```python
from build123d import *

# Parameters (mm, degrees)
SKETCH1_W          = 10
SKETCH1_H          = 54
BASE_FLANGE1_DEPTH = 0.5
EDGE_FLANGE1_DEPTH = 54
CUT_EXTRUDE1_DEPTH = 10
EDGE_FLANGE2_DEPTH = 19.2634
SKETCH11_R         = 1.8
CUT_EXTRUDE2_DEPTH = 10
SKETCH12_R         = 2
CUT_EXTRUDE3_DEPTH = 10


# Sheet-metal steps are written as plain solids
with BuildPart() as part:
    # Sketch1 → Base-Flange1 (new body)
    with BuildSketch(Plane(origin=(0, 0, 0), x_dir=(1, 0, 0), z_dir=(0, 1, 0))):
        with Locations((-31.456172324, -6.536484397)):
            Rectangle(SKETCH1_W, SKETCH1_H)
    extrude(amount=-BASE_FLANGE1_DEPTH)

    # Edge-Flange1 section (across the edge) → Edge-Flange1 (add)
    with BuildSketch(Plane(origin=(-37.192772324, -0.5, 33.536484397), x_dir=(1, 0, 0), z_dir=(0, 0, -1))):
        with BuildLine():
            Line((-0.5, 0.7366), (-0.5, 20))
            Line((-0.5, 20), (0, 20))
            Line((0, 20), (0, 0.7366))
            ThreePointArc((0, 0.7366), (0.215745145, 0.215745145), (0.7366, 0))
            Line((0.7366, 0), (0.7366, -0.5))
            ThreePointArc((0.7366, -0.5), (-0.137808246, -0.137808246), (-0.5, 0.7366))
        make_face()
    extrude(amount=EDGE_FLANGE1_DEPTH)

    # Sketch7 → Cut-Extrude1 (cut)
    with BuildSketch(Plane.ZY.offset(37.692772324)):
        Polygon((-20.463515603, -20.5), (33.536484397, -1.2366), (33.536484397, -20.5), align=None)
    extrude(amount=-CUT_EXTRUDE1_DEPTH, mode=Mode.SUBTRACT)

    # Edge-Flange2 section (across the edge) → Edge-Flange2 (add)
    with BuildSketch(Plane(origin=(-37.192772324, -20.5, -21.200115603), x_dir=(0, 0, 1), z_dir=(0, 1, 0))):
        with BuildLine():
            Line((-0.5, 0.7366), (-0.5, 10))
            Line((-0.5, 10), (0, 10))
            Line((0, 10), (0, 0.7366))
            ThreePointArc((0, 0.7366), (0.215745145, 0.215745145), (0.7366, 0))
            Line((0.7366, 0), (0.7366, -0.5))
            ThreePointArc((0.7366, -0.5), (-0.137808246, -0.137808246), (-0.5, 0.7366))
        make_face()
    extrude(amount=EDGE_FLANGE2_DEPTH)

    # Sketch11 → Cut-Extrude2 (cut)
    with BuildSketch(Plane(origin=(0, 0, -21.700115603), x_dir=(-1, 0, 0), z_dir=(0, 0, -1))):
        with Locations((31.456172324, -6.2366)):
            Circle(SKETCH11_R)
        with Locations((31.456172324, -16.2366)):
            Circle(SKETCH11_R)
    extrude(amount=-CUT_EXTRUDE2_DEPTH, mode=Mode.SUBTRACT)

    # Sketch12 → Cut-Extrude3 (cut)
    with BuildSketch(Plane(origin=(0, 0, 0), x_dir=(1, 0, 0), z_dir=(0, 1, 0))):
        with Locations(Location((-32.456172324, -29.536484397, 0), (0, 0, 270))):
            Circle(SKETCH12_R)
        with Locations(Location((-32.456172324, 15.963515603, 0), (0, 0, 270))):
            Circle(SKETCH12_R)
    extrude(amount=-CUT_EXTRUDE3_DEPTH, mode=Mode.SUBTRACT)


solid = part.part
```
Design review of the part built by this model. Coordinates are the model's own, in mm. A direction names the side the tool comes from. Round coordinates to 2 decimals unless told otherwise and drop trailing zeros. Write each loop counter-clockwise with the first axis right and the second up, starting at its lowest first coordinate (ties: lowest second). Pieces come first, ordered by that corner, then holes. Notation, with made-up numbers: (78.25, 58.25) -> (108.25, 58.25) arc R21 ccw to (108.25, 70.25) -> close; hole circle Ø3 at (-11.75, 7). An arc over 180 degrees is marked (long way). Write item = value, one per line. Start each with the question number.
1) Tool access review of faces 1 (the face through (-37.193, -7, -5)), 2 (the face through (-32, -11, -21.2)), 3 (the face through (-32, -0.5, 6)), 4 (the face through (-32.4, -20.5, -21.5)), 5 (the face through (-37.446, -11.003, 6.158)): name each direction out of +Z, -Z, +X, -X, +Y, -Y from which nothing blocks a thin tool from reaching the whole face with its end or side.
2) Take a section at A-A, the plane x = -35.5. State the section outline as (y, z) points, plus the area to 3 significant figures.
3) Clearance check with flat-ended pins moving along their axes: pin 1 (3 mm diameter, centred on x = -32, z = -13.5, fed in from -Y); pin 2 (4.5 mm diameter, centred on x = -31.46, y = -6.24, fed in from +Z); pin 3 (3 mm diameter, centred on y = -3, z = -12, fed in from +X). State where each tip first meets the part, or that it passes through.
4) Take a section at D-D, the plane z = 11. State the section outline as (x, y) points, plus the area to 3 significant figures.
5) Wall thickness on probe 1 along Y at (x, z) = (-30, -16); probe 2 along X at (y, z) = (-1.5, -19); probe 3 along Z at (x, y) = (-31.5, -12): over which ranges is each line inside the solid? List them lowest first. Write a range as from..to.
6) Take a section at C-C, the plane y = -7. State the section outline as (x, z) points.
7) Mouldability with a two-part tool opening along Y and no side actions: class faces 6 (the face through (-32, 0, 6)), 7 (the face through (-29.658, -16.157, -21.454)), 8 (the face through (-37.34, -11, -21.33)), 9 (the face through (-29.658, -6.157, -21.454)) as +Y half, -Y half, draft (parallel to the pull), parting line (faces both ways), or undercut.
8) Take a section at B-B, the plane x = -31.5. State the section outline as (y, z) points, plus the area to 3 significant figures.
Results list:
q1.face_1 = +Z, +X, -Y
q1.face_2 = +Z, +X, +Y, -Y
q1.face_3 = +Z, -Z, +X, -Y
q1.face_4 = +Z, -Z, +X, -X, -Y
q1.face_5 = +Z, +X, -X, -Y
q2.outline = (-20.5, -21.7) -> (-1.24, -21.7) -> (-1.24, -21.2) -> (-20.5, -21.2) -> close; (-0.5, -20.46) -> (0, -20.46) -> (0, 33.54) -> (-0.5, 33.54) -> close
q2.area = 36.6 mm²
q3.pin_1 = -0.5
q3.pin_2 = -21.2
q3.pin_3 = -37.19
q4.outline = (-37.69, -9.28) -> (-37.19, -9.28) -> (-37.19, -1.24) arc R0.74 cw to (-36.46, -0.5) -> (-26.46, -0.5) -> (-26.46, 0) -> (-36.46, 0) arc R1.24 ccw to (-37.69, -1.24) -> close
q4.area = 9.79 mm²
q5.probe_1 = -0.5..0
q5.probe_2 = -37.69..-37.19
q5.probe_3 = -21.7..-21.2
q6.outline = (-37.69, -20.46) arc R1.24 ccw to (-36.46, -21.7) -> (-33.09, -21.7) -> (-33.09, -21.2) -> (-36.46, -21.2) arc R0.74 cw to (-37.19, -20.46) -> (-37.19, 17.38) -> (-37.69, 17.38) -> close; (-29.83, -21.7) -> (-27.19, -21.7) -> (-27.19, -21.2) -> (-29.83, -21.2) -> close
q7.face_6 = +Y half
q7.face_7 = undercut
q7.face_8 = draft
q7.face_9 = undercut
q8.outline = (-20.5, -21.7) -> (-18.04, -21.7) -> (-18.04, -21.2) -> (-20.5, -21.2) -> close; (-14.44, -21.7) -> (-8.04, -21.7) -> (-8.04, -21.2) -> (-14.44, -21.2) -> close; (-4.44, -21.7) -> (-1.24, -21.7) -> (-1.24, -21.2) -> (-4.44, -21.2) -> close; (-0.5, -20.46) -> (0, -20.46) -> (0, -17.72) -> (-0.5, -17.72) -> close; (-0.5, -14.21) -> (0, -14.21) -> (0, 27.78) -> (-0.5, 27.78) -> close; (-0.5, 31.29) -> (0, 31.29) -> (0, 33.54) -> (-0.5, 33.54) -> close
q8.area = 29.5 mm²
